from build123d import *

# Parameters (mm, degrees)
SKIZZE1_W                       = 120
SKIZZE1_H                       = 50
AUFSATZ_LINEAR_AUSTRAGEN1_DEPTH = 10
SKIZZE3_W                       = 22
SKIZZE3_H                       = 30
SCHNITT_LINEAR_AUSTRAGEN1_DEPTH = 66.76473219
SKIZZE4_W                       = 120
SKIZZE4_H                       = 10
AUFSATZ_LINEAR_AUSTRAGEN2_DEPTH = 10


with BuildPart() as part:
    # Skizze1 → Aufsatz-Linear austragen1 (new body)
    with BuildSketch(Plane(origin=(0, 0, 0), x_dir=(1, 0, 0), z_dir=(0, 1, 0))):
        Rectangle(SKIZZE1_W, SKIZZE1_H)
    extrude(amount=AUFSATZ_LINEAR_AUSTRAGEN1_DEPTH)

    # Skizze3 → Schnitt-Linear austragen1 (cut, through all)
    with BuildSketch(Plane(origin=(0, 10, 0), x_dir=(1, 0, 0), z_dir=(0, 1, 0))):
        with Locations((-35, 0)):
            Rectangle(SKIZZE3_W, SKIZZE3_H)
    extrude(amount=-SCHNITT_LINEAR_AUSTRAGEN1_DEPTH, mode=Mode.SUBTRACT)

    # Skizze4 → Aufsatz-Linear austragen2 (add)
    with BuildSketch(Plane(origin=(0, 10, 0), x_dir=(1, 0, 0), z_dir=(0, 1, 0))):
        with Locations((0, 30)):
            Rectangle(SKIZZE4_W, SKIZZE4_H)
    extrude(amount=-AUFSATZ_LINEAR_AUSTRAGEN2_DEPTH)


solid = part.part
Source: CAD feature listing. Evaluate the final solid. Frame: model axes, mm. A direction names the side the tool comes from. Give positions to 0.01 mm unless a question says otherwise; leave off trailing zeros. Write each loop counter-clockwise with the first axis right and the second up, starting at its lowest first coordinate (ties: lowest second). Pieces come first, ordered by that corner, then holes. Notation, with made-up numbers: (-7.75, 46) - (37.25, 46) arc R29 cw to (37.25, 74) - close; hole circle Ø4 at (-36.75, 53.25). An arc over 180 degrees is marked (long way). Write item = value, one per line. Start each with the question number.
Q1. Cut plane B-B, the plane z = -7.5. Return loops of the section in (x, y), then the cut area to 3 significant figures.
Q2. Pin query (flat end, axial travel): pin 1 Ø4 at (x, z) = (-37, -24.5) entering from -Y. Return the tip coordinate at first contact, or that it passes through.
Q3. Draft query along Z for faces 3 (the flat face through (-1, 5, 25)), 4 (the flat face through (-1, 5, -35)), 5 (the flat face through (-24, 5, 0)). Return one class per face: +Z half, -Z half, draft (parallel to the pull), parting line (faces both ways), or undercut.
Q4. Reachability of faces 1 (the flat face through (-35, 5, 15)), 2 (the flat face through (-1, 0, -5)) from +Z, -Z, +X, -X, +Y, -Y: full face, straight path, thin tool, end or side. Return the list, or none.
Q5. Cut plane C-C, the plane y = 5.75. Return loops of the section in (x, z), then the cut area to 3 significant figures.
Q6. Cut plane A-A, the plane x = -42.5. Return loops of the section in (y, z), then the cut area to 3 significant figures.
Q7. Material intervals for probe 1 along X at (y, z) = (4.25, -11); probe 2 along Z at (x, y) = (-25, 7), sorted ascending.
Computed values:
q1.outline = (-60, 0) - (-46, 0) - (-46, 10) - (-60, 10) - close; (-24, 0) - (60, 0) - (60, 10) - (-24, 10) - close
q1.area = 980 mm²
q2.pin_1 = 0
q3.face_3 = +Z half
q3.face_4 = -Z half
q3.face_5 = undercut
q4.face_1 = +Y, -Y
q4.face_2 = +Z, -Z, +X, -X, -Y
q5.outline = (-60, -35) - (60, -35) - (60, 25) - (-60, 25) - close; hole (-46, -15) - (-24, -15) - (-24, 15) - (-46, 15) - close
q5.area = 6,540 mm²
q6.outline = (0, -35) - (10, -35) - (10, -15) - (0, -15) - close; (0, 15) - (10, 15) - (10, 25) - (0, 25) - close
q6.area = 300 mm²
q7.probe_1 = -60 to -46, -24 to 60
q7.probe_2 = -35 to -15, 15 to 25
